Can you work these out from the model? Positions are in its coordinate system, mm. Give positions to 0.01 mm unless a question says otherwise; leave off trailing zeros. Write each loop counter-clockwise with the first axis right and the second up, starting at its lowest first coordinate (ties: lowest second). Pieces come first, ordered by that corner, then holes.
Autodesk Fusion 360 part; units mm, degrees
sketch "movingPlatform" plane through (0, 0, 0) normal (0, 0, 1) x (1, 0, 0)
  line L0 (-75, 59) -> (75, 59)
  line L1 (75, 59) -> (75, -59)
  line L2 (75, -59) -> (-75, -59)
  line L3 (-75, -59) -> (-75, 59)
  line L4 (-75, 59) -> (75, -59) construction
  line L5 (75, 59) -> (-75, -59) construction
  circle A0 centre (-60, -34) radius 6.45
  line L6 (0, 2.5) -> (0, 20)
  circle A1 centre (60, -34) radius 6.45
  circle A2 centre (0, 34) radius 6.45
  circle A3 centre (-46, -46) radius 1.588
  circle A4 centre (-15.5, -15.5) radius 1.588
  circle A5 centre (0, 0) radius 57 construction
  circle A6 centre (15.5, -15.5) radius 1.588
  circle A7 centre (15.5, 15.5) radius 1.588
  circle A8 centre (46, -46) radius 1.588
  circle A9 centre (-46, 46) radius 1.588
  circle A10 centre (46, 46) radius 1.588
  circle A11 centre (-15.5, 15.5) radius 1.588
  circle A12 centre (0, 0) radius 1.588
  dimension "d1" = 150
  dimension "d2" = 118
  dimension "d3" = 12.9
  dimension "d4" = 120
  dimension "d6" = 68
  dimension "d7" = 25
  dimension "d8" = 25
  dimension "d9" = 3.176
  dimension "d12" = 92
  dimension "d13" = 92
  dimension "d21" = 3.176
  dimension "d24" = 31
  dimension "d25" = 31
  dimension "d27" = 15.5
  dimension "d31" = 114
  dimension "d34" = 46
  dimension "d37" = 46
  dimension "d49" = 15.5
  dimension "d52" = 12.9
  dimension "d53" = 12.9
  dimension "d56" = 3.176
extrude "Extrude3" add sketch "movingPlatform" along normal blind 3.8
equation "d4 = 132.800 mm - 12.8 mm"
(1) If I drill on L1, parallel to Y at x = 46, z = 2.9; L2, parallel to X at y = -34.5, z = 1.9; L3, parallel to Y at x = 0, z = 2.8, over which ranges is the centre line in solid material (lowest first)?
Returned:
L1: y = -59 to -47.59, -44.41 to 44.41, 47.59 to 59
L2: x = -75 to -66.43, -53.57 to 53.57, 66.43 to 75
L3: y = -59 to -1.59, 1.59 to 27.55, 40.45 to 59
(2) Will these pins go through, and if not, where does the flat tip stop? P1, Ø3.5, axis at x = -15.5, y = 15.5, coming from the -Z side; P2, Ø1.9, axis at x = -46, y = -46, coming from the -Z side.
Returned:
P1: stops at z = 0
P2: passes through
(3) Imagine slicing it at B-B, the plane z = 2.9. Give the number of separate pieces and of enclosed holes in the cut face, plus the area to 3 significant figures.
Returned:
separate pieces: 1
enclosed holes: 12
area: 17,200 mm2
(4) Imagine slicing it at A-A, the plane x = 15.5. Write out the boundary of the cut face in (y, z), plus the area to 3 significant figures.
Returned:
outline: (-59, 0) - (-17.09, 0) - (-17.09, 3.8) - (-59, 3.8) - close; (-13.91, 0) - (13.91, 0) - (13.91, 3.8) - (-13.91, 3.8) - close; (17.09, 0) - (59, 0) - (59, 3.8) - (17.09, 3.8) - close
area: 424 mm2
(5) If we mould it in two halves opening along X, with no side actions, what happens to faces 1 (the face through (-60.8, -40.4, 1.9)), 2 (the face through (-1, -12, 3.8)), 3 (the face through (-75, -1, 2))? For each: +X half, -X half, draft (parallel to the pull), parting line (faces both ways), or undercut.
Returned:
face 1: undercut
face 2: draft
face 3: -X half
(6) Imagine slicing it at C-C, the plane y = -15.5. Write out the boundary of the cut face in (x, z).
Returned:
outline: (-75, 0) - (-17.09, 0) - (-17.09, 3.8) - (-75, 3.8) - close; (-13.91, 0) - (13.91, 0) - (13.91, 3.8) - (-13.91, 3.8) - close; (17.09, 0) - (75, 0) - (75, 3.8) - (17.09, 3.8) - close
